```python
from build123d import *

# Parameters (mm, degrees)
F0_R     = 1.5
F1_DEPTH = 1.5
F2_R     = 5


with BuildPart() as f1:
    # F0 (on Top) → F1 (new body)
    with BuildSketch(Plane.XY):
        Polygon((-25.455844, 39.59798), (-39.59798, 25.455844), (-26, 11.857864), (-26, -11.857864), (-39.59798, -25.455844), (-25.455844, -39.59798), (-15.857864, -30), (15.857864, -30), (25.455844, -39.59798), (39.59798, -25.455844), (26, -11.857864), (26, 11.857864), (39.59798, 25.455844), (25.455844, 39.59798), (15.857864, 30), (-15.857864, 30), align=None)
        with Locations((-25.149495, -33.634776)):
            Circle(F0_R, mode=Mode.SUBTRACT)
        with Locations((-33.634776, -25.149495)):
            Circle(F0_R, mode=Mode.SUBTRACT)
        with Locations((-15.25, -15.25)):
            Circle(F0_R, mode=Mode.SUBTRACT)
        with Locations((25.149495, -33.634776)):
            Circle(F0_R, mode=Mode.SUBTRACT)
        with Locations((33.634776, -25.149495)):
            Circle(F0_R, mode=Mode.SUBTRACT)
        with Locations((15.25, -15.25)):
            Circle(F0_R, mode=Mode.SUBTRACT)
        with BuildLine():
            ThreePointArc((-22.5, 10.5), (-21.25, 11.75), (-20, 10.5))
            Line((-20, 10.5), (-20, -10.5))
            ThreePointArc((-20, -10.5), (-21.25, -11.75), (-22.5, -10.5))
            Line((-22.5, -10.5), (-22.5, 10.5))
        make_face(mode=Mode.SUBTRACT)
        with Locations((-15.25, 15.25)):
            Circle(F0_R, mode=Mode.SUBTRACT)
        with Locations((-33.634776, 25.149495)):
            Circle(F0_R, mode=Mode.SUBTRACT)
        with Locations((-25.149495, 33.634776)):
            Circle(F0_R, mode=Mode.SUBTRACT)
        with Locations((15.25, 15.25)):
            Circle(F0_R, mode=Mode.SUBTRACT)
        with BuildLine():
            Line((20, -10.5), (20, 10.5))
            ThreePointArc((20, 10.5), (21.25, 11.75), (22.5, 10.5))
            Line((22.5, 10.5), (22.5, -10.5))
            ThreePointArc((22.5, -10.5), (21.25, -11.75), (20, -10.5))
        make_face(mode=Mode.SUBTRACT)
        with Locations((33.634776, 25.149495)):
            Circle(F0_R, mode=Mode.SUBTRACT)
        with Locations((25.149495, 33.634776)):
            Circle(F0_R, mode=Mode.SUBTRACT)
    extrude(amount=F1_DEPTH)

    # F2
    f2_edges = [f1.edges().sort_by_distance(p)[0] for p in [
        (-15.857864, 30, 0.75),
        (15.857864, 30, 0.75),
        (26, 11.857864, 0.75),
        (26, -11.857864, 0.75),
        (-26, -11.857864, 0.75),
        (-26, 11.857864, 0.75),
        (-15.857864, -30, 0.75),
        (15.857864, -30, 0.75),
    ]]
    fillet(f2_edges, radius=F2_R)


solid = f1.part
```
Read the model definition and answer for the solid it produces. Units are mm, in the model's axes. A direction names the side the tool comes from. Give positions to 0.01 mm unless a question says otherwise; leave off trailing zeros. Order: outer loops, then holes, each group sorted by start corner. A loop starts at its lowest first (then second) coordinate and runs counter-clockwise, first axis right, second up. Notation, with made-up numbers: (40, -5.5) -> (69, -5.5) arc R28 ccw to (69, 31.5) -> close; hole circle Ø3 at (89.5, 52). An arc over 180 degrees is marked (long way). Write item = value, one per line.
1. A cutting plane is placed at C-C, the plane x = -4.5. Write down the section's boundary in (y, z).
Numbers:
outline = (-30, 0) -> (30, 0) -> (30, 1.5) -> (-30, 1.5) -> close
2. For faces 4 (the face through (33.616, -19.474, 0.74)), 5 (the face through (-23.764, -34.209, 0.74)), 6 (the face through (-21.45, -35.59, 0.74)), 7 (the face through (-33.616, 19.474, 0.74)), determine the directions among +Z, -Z, +X, -X, +Y, -Y from which every point of the face is accessible in a straight line to the end or side of a thin tool.
Numbers:
face_4 = +Z, -Z, +X
face_5 = +Z, -Z
face_6 = +Z, -Z, -Y
face_7 = +Z, -Z, -X
3. A cutting plane is placed at B-B, the plane x = -15.25. Write down the section's boundary in (y, z).
Numbers:
outline = (-30.22, 0) -> (-16.75, 0) -> (-16.75, 1.5) -> (-30.22, 1.5) -> close; (-13.75, 0) -> (13.75, 0) -> (13.75, 1.5) -> (-13.75, 1.5) -> close; (16.75, 0) -> (30.22, 0) -> (30.22, 1.5) -> (16.75, 1.5) -> close
4. A cutting plane is placed at D-D, the plane z = 0.65. Count the separate pieces of the cut face and the enclosed holes in it, and give its area (3 significant figures).
Numbers:
separate_pieces = 1
enclosed_holes = 14
area = 3,870 mm²
5. Straight lines are drawn through the part: line 1 along X through (y, z) = (0.5, 1.05); line 2 along X through (y, z) = (-25, 0.1); line 3 along Y through (x, z) = (-16, 0.15). For each, find the intervals that lie inside material, in ascending order.
Numbers:
line_1 = -26 to -22.5, -20 to 20, 22.5 to 26
line_2 = -39.14 to -35.13, -32.14 to 32.14, 35.13 to 39.14
line_3 = -30.52 to -16.55, -13.95 to 13.95, 16.55 to 30.52
6. A cutting plane is placed at A-A, the plane y = -6.5. Write down the section's boundary in (x, z).
Numbers:
outline = (-26, 0) -> (-22.5, 0) -> (-22.5, 1.5) -> (-26, 1.5) -> close; (-20, 0) -> (20, 0) -> (20, 1.5) -> (-20, 1.5) -> close; (22.5, 0) -> (26, 0) -> (26, 1.5) -> (22.5, 1.5) -> close
7. Given pin 1 (4 mm diameter, centred on x = -15.25, y = -15.25, fed in from -Z); pin 2 (0.8 mm diameter, centred on y = 3.5, z = 1, fed in from -X), each flat-ended and moving along its own axis, determine where each tip first touches the part or whether it passes through.
Numbers:
pin_1 = 0
pin_2 = -26
8. The mould has two halves that part along Y. Classify faces 1 (the face through (-1, 1, 0)), 2 (the face through (-32.626, -32.428, 0.74)), 3 (the face through (34.33, 23.82, 0.74)): +Y half, -Y half, draft (parallel to the pull), parting line (faces both ways), or undercut.
Numbers:
face_1 = draft
face_2 = -Y half
face_3 = undercut
